Build history of the part. All positions in model axes, mm. Face numbers are marked on the shaded views. A direction names the side the tool comes from. Round coordinates to 2 decimals unless told otherwise and drop trailing zeros. Write each loop counter-clockwise with the first axis right and the second up, starting at its lowest first coordinate (ties: lowest second). Pieces come first, ordered by that corner, then holes.
Item 1: Band-saw the part on B-B, the plane z = 0. Write the cut outline in (x, y) (3 decimals), then the cut area to 4 significant figures.
Item 2: Band-saw the part on A-A, the plane x = 0. Write the cut outline in (y, z) (3 decimals), then the cut area to 4 significant figures.
Item 3: Mould opens along X. For the marked faces 1, 2 and 3 say: +X half, -X half, draft (parallel to the pull), parting line (faces both ways), or undercut.
Item 4: 3-axis set-ups, long thin cutter, end or side, ignore diameter. For the marked faces 4, 5, 6 and 7: which of +Z, -Z, +X, -X, +Y, -Y reach the whole face in a straight line?
Item 5: Drop flat-ended pins along their axis: pin 1 Ø1.5 at (y, z) = (1, 11) entering from -X; pin 2 Ø1.5 at (y, z) = (2.5, 7.5) entering from -X. Give the stop position or say it passes through.
Item 6: Wall check: probe 1 along Z at (x, y) = (14.5, 1.9); probe 2 along X at (y, z) = (0.7, -13.5); probe 3 along Z at (x, y) = (13, 0.6). Give the ranges that are in metal, low to high.
Item 7: Band-saw the part on D-D, the plane z = 9. Write the cut outline in (x, y).
Item 8: Band-saw the part on C-C, the plane z = -5.5. Write the cut outline in (x, y), then the cut area to 3 significant figures.
```python
from build123d import *

# Parameters (mm, degrees)
SKETCH1_R           = 16.5
BOSS_EXTRUDE1_DEPTH = 3
CUT_EXTRUDE1_DEPTH  = 4
CIRPATTERN1_COUNT   = 20
SKETCH4_R           = 1.5
CUT_EXTRUDE3_DEPTH  = 10


with BuildPart() as part:
    # Sketch1 → Boss-Extrude1 (new body)
    with BuildSketch(Plane(origin=(0, 0, 0), x_dir=(1, 0, 0), z_dir=(0, 1, 0))):
        Circle(SKETCH1_R)
    extrude(amount=BOSS_EXTRUDE1_DEPTH)

    # Sketch2 → Cut-Extrude1 (cut, through all)
    with BuildSketch(Plane(origin=(0, 3, 0), x_dir=(1, 0, 0), z_dir=(0, 1, 0))):
        with BuildLine():
            ThreePointArc((-0.661599664, 13.108314571), (0, 13.125), (0.661599664, 13.108314571))
            ThreePointArc((0.661599664, 13.108314571), (1.127215597, 14.845961564), (2.087005275, 16.367480227))
            ThreePointArc((2.087005275, 16.367480227), (0, 16.5), (-2.087005275, 16.367480227))
            ThreePointArc((-2.087005275, 16.367480227), (-1.127215597, 14.845961564), (-0.661599664, 13.108314571))
        make_face()
    cut_extrude1 = extrude(amount=-CUT_EXTRUDE1_DEPTH, mode=Mode.SUBTRACT)

    # CirPattern1: Cut-Extrude1 ×20 about axis
    cirpattern1_axis = Axis((0, 0, 0), (0, 1, 0))
    for i in range(1, CIRPATTERN1_COUNT):
        add(cut_extrude1.rotate(cirpattern1_axis, i * 360 / CIRPATTERN1_COUNT), mode=Mode.SUBTRACT)

    # Sketch4 → Cut-Extrude3 (cut)
    with BuildSketch(Plane.XZ):
        Circle(SKETCH4_R)
    extrude(amount=-CUT_EXTRUDE3_DEPTH, mode=Mode.SUBTRACT)


solid = part.part
```
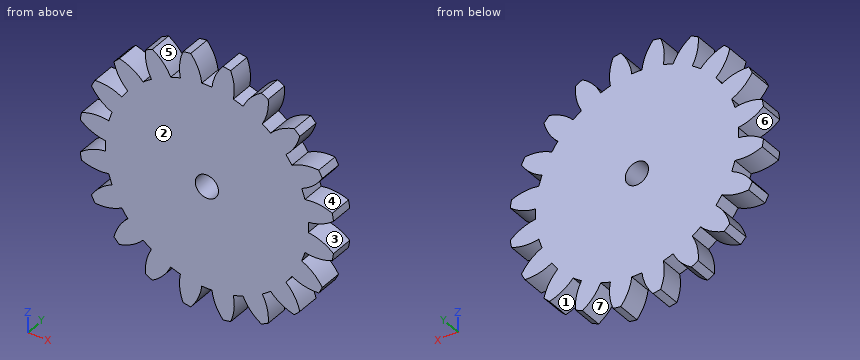
Results:
1. outline: (-13.125, 0) - (-1.5, 0) - (-1.5, 3) - (-13.125, 3) - close; (1.5, 0) - (13.125, 0) - (13.125, 3) - (1.5, 3) - close
1. area: 69.75 mm2
2. outline: (0, -13.125) - (3, -13.125) - (3, -1.5) - (0, -1.5) - close; (0, 1.5) - (3, 1.5) - (3, 13.125) - (0, 13.125) - close
2. area: 69.75 mm2
3. face 1: undercut
3. face 2: draft
3. face 3: +X half
4. face 4: +Y, -Y
4. face 5: +Z, +Y, -Y
4. face 6: -X, +Y, -Y
4. face 7: -Z, +Y, -Y
5. pin 1: stops at x = -12.01
5. pin 2: stops at x = -14.92
6. probe 1: z = -7.87 to -6.43, -3.51 to -0.99, 0.99 to 3.51, 6.43 to 7.87
6. probe 2: x = -7.94 to -5.43, -3.53 to -0.72, 0.72 to 3.53, 5.43 to 7.94
6. probe 3: z = -7.88 to -5.08, -3.48 to 3.48, 5.08 to 7.88
7. outline: (-10.92, 0) - (10.92, 0) - (10.92, 3) - (-10.92, 3) - close
8. outline: (-13.58, 0) - (13.58, 0) - (13.58, 3) - (-13.58, 3) - close
8. area: 81.5 mm2
